Geometry: final body of the model. Coordinates: model frame, mm. Round coordinates to 2 decimals unless told otherwise and drop trailing zeros. Loops run counter-clockwise (first coordinate to the right, second up) from the corner with the lowest first, then second, coordinate; pieces in that order, holes last. Notation, with made-up numbers: M 65.25,60 L 72.25,60 A31 ccw 72.25,85 Z; hole C -24,66 d10. An arc over 180 degrees is marked long. Answer as a JSON object with one key per item and string values.
from build123d import *

# Parameters (mm, degrees)
BOSS_EXTRUDE1_DEPTH = 4
SKETCH3_W           = 650
SKETCH3_H           = 650
SKETCH3_W_2         = 2250
SKETCH3_H_2         = 490
CUT_EXTRUDE1_DEPTH  = 1458.743461656


with BuildPart() as part:
    # Sketch1 → Boss-Extrude1 (new body)
    with BuildSketch(Plane.XY):
        Polygon((-1250, 750), (0, 750), (1250, 750), (1250, -750), (-1250, -750), align=None)
    extrude(amount=BOSS_EXTRUDE1_DEPTH)

    # Sketch3 → Cut-Extrude1 (cut, through all)
    with BuildSketch(Plane.XY.offset(4)):
        with Locations((-775, 286)):
            Rectangle(SKETCH3_W, SKETCH3_H)
        with Locations((775, 286)):
            Rectangle(SKETCH3_W, SKETCH3_H)
        with Locations((0, -434)):
            Rectangle(SKETCH3_W_2, SKETCH3_H_2)
    extrude(amount=-CUT_EXTRUDE1_DEPTH, mode=Mode.SUBTRACT)


solid = part.part
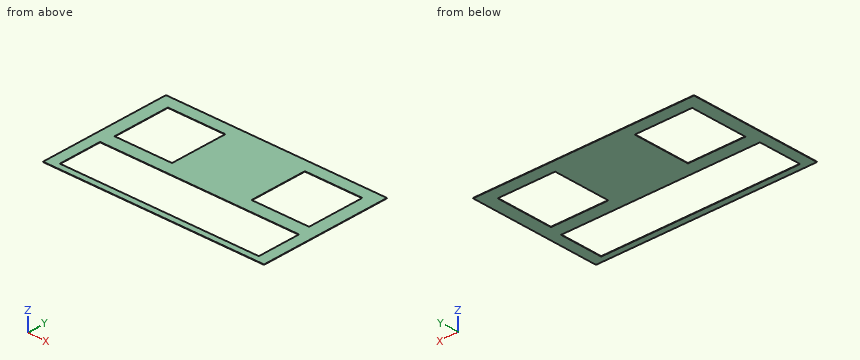
1) Ray query, line 1 (Y direction, x = -822, z = 3.15); line 2 (X direction, y = 345, z = 1.65); line 3 (Y direction, x = 136.5, z = 3.45). Return the intervals inside material, ascending.
Results:
{"line 1": "-750 to -679, -189 to -39, 611 to 750", "line 2": "-1250 to -1100, -450 to 450, 1100 to 1250", "line 3": "-750 to -679, -189 to 750"}
2) Section query B-B (x = -743). Return the cut outline in (y, z).
Results:
{"outline": "M -750,0 L -679,0 L -679,4 L -750,4 Z; M -189,0 L -39,0 L -39,4 L -189,4 Z; M 611,0 L 750,0 L 750,4 L 611,4 Z"}
3) Section query C-C (y = -626). Return the cut outline in (x, z), and give its area (3 significant figures).
Results:
{"outline": "M -1250,0 L -1125,0 L -1125,4 L -1250,4 Z; M 1125,0 L 1250,0 L 1250,4 L 1125,4 Z", "area": "1,000 mm2"}
4) Section query A-A (z = 3.15). Return the cut outline in (x, y).
Results:
{"outline": "M -1250,-750 L 1250,-750 L 1250,750 L -1250,750 Z; hole M -1125,-679 L 1125,-679 L 1125,-189 L -1125,-189 Z; hole M -1100,-39 L -450,-39 L -450,611 L -1100,611 Z; hole M 450,-39 L 1100,-39 L 1100,611 L 450,611 Z"}
5) Section query D-D (x = -225.5). Return the cut outline in (y, z), and give its area (3 significant figures).
Results:
{"outline": "M -750,0 L -679,0 L -679,4 L -750,4 Z; M -189,0 L 750,0 L 750,4 L -189,4 Z", "area": "4,040 mm2"}
